```python
from build123d import *

# Parameters (mm, degrees)
CROQUIS1_W              = 440
CROQUIS1_H              = 440
SALIENTE_EXTRUIR1_DEPTH = 9
CROQUIS2_R              = 2
CORTAR_EXTRUIR1_DEPTH   = 312.257128432
CORTAR_EXTRUIR2_DEPTH   = 312.257128432
CORTAR_EXTRUIR3_DEPTH   = 312.257128432
REDONDEO1_R             = 5
CROQUIS5_R              = 2
CORTAR_EXTRUIR4_DEPTH   = 312.257128432
SALIENTE_EXTRUIR3_DEPTH = 9
CROQUIS8_R              = 1.5
CORTAR_EXTRUIR7_DEPTH   = 334.138109498
CROQUIS9_R              = 3
CORTAR_EXTRUIR8_DEPTH   = 334.138109498


with BuildPart() as part:
    # Croquis1 → Saliente-Extruir1 (new body)
    with BuildSketch(Plane(origin=(0, 0, 0), x_dir=(1, 0, 0), z_dir=(0, 1, 0))):
        Rectangle(CROQUIS1_W, CROQUIS1_H)
    extrude(amount=SALIENTE_EXTRUIR1_DEPTH)

    # Croquis2 → Cortar-Extruir1 (cut, through all)
    with BuildSketch(Plane(origin=(0, 9, 0), x_dir=(1, 0, 0), z_dir=(0, 1, 0))):
        with Locations(Location((-210, 210, 0), (0, 0, 270))):
            Circle(CROQUIS2_R)
        with Locations(Location((0, 210, 0), (0, 0, 270))):
            Circle(CROQUIS2_R)
        with Locations(Location((-210, 190, 0), (0, 0, 270))):
            Circle(CROQUIS2_R)
        with Locations(Location((-10, 190, 0), (0, 0, 270))):
            Circle(CROQUIS2_R)
        with Locations(Location((-210, 0, 0), (0, 0, 270))):
            Circle(CROQUIS2_R)
        with Locations(Location((-10, 0, 0), (0, 0, 270))):
            Circle(CROQUIS2_R)
        with Locations(Location((0, -210, 0), (0, 0, 90))):
            Circle(CROQUIS2_R)
        with Locations(Location((-10, -190, 0), (0, 0, 90))):
            Circle(CROQUIS2_R)
        with Locations(Location((-210, -190, 0), (0, 0, 90))):
            Circle(CROQUIS2_R)
        with Locations(Location((-210, -210, 0), (0, 0, 90))):
            Circle(CROQUIS2_R)
        with Locations(Location((10, -190, 0), (0, 0, 270))):
            Circle(CROQUIS2_R)
        with Locations(Location((210, -210, 0), (0, 0, 270))):
            Circle(CROQUIS2_R)
        with Locations(Location((210, -190, 0), (0, 0, 270))):
            Circle(CROQUIS2_R)
        with Locations(Location((210, 0, 0), (0, 0, 90))):
            Circle(CROQUIS2_R)
        with Locations(Location((10, 0, 0), (0, 0, 90))):
            Circle(CROQUIS2_R)
        with Locations(Location((10, 190, 0), (0, 0, 90))):
            Circle(CROQUIS2_R)
        with Locations(Location((210, 190, 0), (0, 0, 90))):
            Circle(CROQUIS2_R)
        with Locations(Location((210, 210, 0), (0, 0, 90))):
            Circle(CROQUIS2_R)
        with Locations(Location((-91.6, 190, 0), (0, 0, 270))):
            Circle(CROQUIS2_R)
        with Locations(Location((91.6, 190, 0), (0, 0, 90))):
            Circle(CROQUIS2_R)
        with Locations(Location((-91.6, 0, 0), (0, 0, 270))):
            Circle(CROQUIS2_R)
        with Locations(Location((91.6, -190, 0), (0, 0, 270))):
            Circle(CROQUIS2_R)
        with Locations(Location((-91.6, -190, 0), (0, 0, 90))):
            Circle(CROQUIS2_R)
        with Locations(Location((91.6, 0, 0), (0, 0, 90))):
            Circle(CROQUIS2_R)
    extrude(amount=-CORTAR_EXTRUIR1_DEPTH, mode=Mode.SUBTRACT)

    # Croquis3 → Cortar-Extruir2 (cut, through all)
    with BuildSketch(Plane(origin=(0, 9, 0), x_dir=(1, 0, 0), z_dir=(0, 1, 0))):
        Polygon((-200, -70), (-200, 70), (-191, 85), (-171, 85), (-162, 70), (-162, -70), (-171, -85), (-191, -85), align=None)
        Polygon((171, 85), (162, 70), (162, -70), (171, -85), (191, -85), (200, -70), (200, 70), (191, 85), align=None)
    extrude(amount=-CORTAR_EXTRUIR2_DEPTH, mode=Mode.SUBTRACT)

    # Croquis4 → Cortar-Extruir3 (cut, through all)
    with BuildSketch(Plane(origin=(0, 9, 0), x_dir=(1, 0, 0), z_dir=(0, 1, 0))):
        with BuildLine():
            Line((160.8, 100), (140.8, 100))
            ThreePointArc((140.8, 100), (112.515728753, 111.715728753), (100.8, 140))
            Line((100.8, 140), (100.8, 160))
            ThreePointArc((100.8, 160), (112.515728753, 188.284271247), (140.8, 200))
            Line((140.8, 200), (160.8, 200))
            ThreePointArc((160.8, 200), (189.084271247, 188.284271247), (200.8, 160))
            Line((200.8, 160), (200.8, 140))
            ThreePointArc((200.8, 140), (189.084271247, 111.715728753), (160.8, 100))
        make_face()
        with BuildLine():
            Line((-160.8, 200), (-140.8, 200))
            ThreePointArc((-140.8, 200), (-112.515728753, 188.284271247), (-100.8, 160))
            Line((-100.8, 160), (-100.8, 140))
            ThreePointArc((-100.8, 140), (-112.515728753, 111.715728753), (-140.8, 100))
            Line((-140.8, 100), (-160.8, 100))
            ThreePointArc((-160.8, 100), (-189.084271247, 111.715728753), (-200.8, 140))
            Line((-200.8, 140), (-200.8, 160))
            ThreePointArc((-200.8, 160), (-189.084271247, 188.284271247), (-160.8, 200))
        make_face()
        with BuildLine():
            Line((-160.8, -100), (-140.8, -100))
            ThreePointArc((-140.8, -100), (-112.515728753, -111.715728753), (-100.8, -140))
            Line((-100.8, -140), (-100.8, -160))
            ThreePointArc((-100.8, -160), (-112.515728753, -188.284271247), (-140.8, -200))
            Line((-140.8, -200), (-160.8, -200))
            ThreePointArc((-160.8, -200), (-189.084271247, -188.284271247), (-200.8, -160))
            Line((-200.8, -160), (-200.8, -140))
            ThreePointArc((-200.8, -140), (-189.084271247, -111.715728753), (-160.8, -100))
        make_face()
        with BuildLine():
            Line((200.8, -160), (200.8, -140))
            ThreePointArc((200.8, -140), (189.084271247, -111.715728753), (160.8, -100))
            Line((160.8, -100), (140.8, -100))
            ThreePointArc((140.8, -100), (112.515728753, -111.715728753), (100.8, -140))
            Line((100.8, -140), (100.8, -160))
            ThreePointArc((100.8, -160), (112.515728753, -188.284271247), (140.8, -200))
            Line((140.8, -200), (160.8, -200))
            ThreePointArc((160.8, -200), (189.084271247, -188.284271247), (200.8, -160))
        make_face()
    extrude(amount=-CORTAR_EXTRUIR3_DEPTH, mode=Mode.SUBTRACT)

    # Redondeo1
    redondeo1_edges = [part.edges().sort_by_distance(p)[0] for p in [
        (-171, 4.5, 85),
        (-191, 4.5, 85),
        (-191, 4.5, -85),
        (-171, 4.5, -85),
        (171, 4.5, -85),
        (191, 4.5, -85),
        (191, 4.5, 85),
        (171, 4.5, 85),
    ]]
    fillet(redondeo1_edges, radius=REDONDEO1_R)

    # Croquis5 → Cortar-Extruir4 (cut, through all)
    with BuildSketch(Plane(origin=(0, 9, 0), x_dir=(1, 0, 0), z_dir=(0, 1, 0))):
        with Locations(Location((-210, 165, 0), (0, 0, 270))):
            Circle(CROQUIS5_R)
        with Locations(Location((-210, 135, 0), (0, 0, 270))):
            Circle(CROQUIS5_R)
        with Locations(Location((-210, -135, 0), (0, 0, 90))):
            Circle(CROQUIS5_R)
        with Locations(Location((-210, -165, 0), (0, 0, 90))):
            Circle(CROQUIS5_R)
        with Locations(Location((210, -165, 0), (0, 0, 270))):
            Circle(CROQUIS5_R)
        with Locations(Location((210, -135, 0), (0, 0, 270))):
            Circle(CROQUIS5_R)
        with Locations(Location((210, 135, 0), (0, 0, 90))):
            Circle(CROQUIS5_R)
        with Locations(Location((210, 165, 0), (0, 0, 90))):
            Circle(CROQUIS5_R)
    extrude(amount=-CORTAR_EXTRUIR4_DEPTH, mode=Mode.SUBTRACT)

    # Croquis7 → Saliente-Extruir3 (add)
    with BuildSketch(Plane(origin=(0, 9, 0), x_dir=(1, 0, 0), z_dir=(0, 1, 0))):
        Polygon((220, 220), (-220, 220), (-190, 250), (190, 250), align=None)
        Polygon((220, -220), (190, -250), (-190, -250), (-220, -220), align=None)
    extrude(amount=-SALIENTE_EXTRUIR3_DEPTH)

    # Croquis8 → Cortar-Extruir7 (cut, through all)
    with BuildSketch(Plane(origin=(0, 9, 0), x_dir=(1, 0, 0), z_dir=(0, 1, 0))):
        with Locations(Location((-75, 242.5, 0), (0, 0, 270))):
            Circle(CROQUIS8_R)
        with Locations(Location((-75, 227.5, 0), (0, 0, 90))):
            Circle(CROQUIS8_R)
        with Locations(Location((75, 227.5, 0), (0, 0, 270))):
            Circle(CROQUIS8_R)
        with Locations(Location((75, 242.5, 0), (0, 0, 90))):
            Circle(CROQUIS8_R)
        with Locations(Location((-186.893398282, 242.5, 0), (0, 0, 270))):
            Circle(CROQUIS8_R)
        with Locations(Location((-204.571067812, 224.82233047, 0), (0, 0, 270))):
            Circle(CROQUIS8_R)
        with Locations(Location((-156.893398282, 242.5, 0), (0, 0, 270))):
            Circle(CROQUIS8_R)
        with Locations(Location((-156.893398282, 227.5, 0), (0, 0, 90))):
            Circle(CROQUIS8_R)
        with Locations(Location((-186.893398282, 227.5, 0), (0, 0, 90))):
            Circle(CROQUIS8_R)
        with Locations(Location((186.893398282, 227.5, 0), (0, 0, 270))):
            Circle(CROQUIS8_R)
        with Locations(Location((156.893398282, 227.5, 0), (0, 0, 270))):
            Circle(CROQUIS8_R)
        with Locations(Location((156.893398282, 242.5, 0), (0, 0, 90))):
            Circle(CROQUIS8_R)
        with Locations(Location((204.571067812, 224.82233047, 0), (0, 0, 90))):
            Circle(CROQUIS8_R)
        with Locations(Location((186.893398282, 242.5, 0), (0, 0, 90))):
            Circle(CROQUIS8_R)
        with Locations(Location((186.893398282, -242.5, 0), (0, 0, 270))):
            Circle(CROQUIS8_R)
        with Locations(Location((204.571067812, -224.82233047, 0), (0, 0, 270))):
            Circle(CROQUIS8_R)
        with Locations(Location((156.893398282, -242.5, 0), (0, 0, 270))):
            Circle(CROQUIS8_R)
        with Locations(Location((156.893398282, -227.5, 0), (0, 0, 90))):
            Circle(CROQUIS8_R)
        with Locations(Location((186.893398282, -227.5, 0), (0, 0, 90))):
            Circle(CROQUIS8_R)
        with Locations(Location((-186.893398282, -227.5, 0), (0, 0, 270))):
            Circle(CROQUIS8_R)
        with Locations(Location((-156.893398282, -227.5, 0), (0, 0, 270))):
            Circle(CROQUIS8_R)
        with Locations(Location((-156.893398282, -242.5, 0), (0, 0, 90))):
            Circle(CROQUIS8_R)
        with Locations(Location((-204.571067812, -224.82233047, 0), (0, 0, 90))):
            Circle(CROQUIS8_R)
        with Locations(Location((-186.893398282, -242.5, 0), (0, 0, 90))):
            Circle(CROQUIS8_R)
    extrude(amount=-CORTAR_EXTRUIR7_DEPTH, mode=Mode.SUBTRACT)

    # Croquis9 → Cortar-Extruir8 (cut, through all)
    with BuildSketch(Plane(origin=(0, 9, 0), x_dir=(1, 0, 0), z_dir=(0, 1, 0))):
        with Locations(Location((-210, 210, 0), (0, 0, 270))):
            Circle(CROQUIS9_R)
        with Locations(Location((-210, 190, 0), (0, 0, 270))):
            Circle(CROQUIS9_R)
        with Locations(Location((-210, 165, 0), (0, 0, 270))):
            Circle(CROQUIS9_R)
        with Locations(Location((-210, 135, 0), (0, 0, 270))):
            Circle(CROQUIS9_R)
        with Locations(Location((-210, 0, 0), (0, 0, 270))):
            Circle(CROQUIS9_R)
        with Locations(Location((-91.6, 0, 0), (0, 0, 270))):
            Circle(CROQUIS9_R)
        with Locations(Location((-10, 0, 0), (0, 0, 270))):
            Circle(CROQUIS9_R)
        with Locations(Location((0, 210, 0), (0, 0, 270))):
            Circle(CROQUIS9_R)
        with Locations(Location((-10, 190, 0), (0, 0, 270))):
            Circle(CROQUIS9_R)
        with Locations(Location((-91.6, 190, 0), (0, 0, 270))):
            Circle(CROQUIS9_R)
        with Locations(Location((210, 0, 0), (0, 0, 90))):
            Circle(CROQUIS9_R)
        with Locations(Location((91.6, 0, 0), (0, 0, 90))):
            Circle(CROQUIS9_R)
        with Locations(Location((10, 0, 0), (0, 0, 90))):
            Circle(CROQUIS9_R)
        with Locations(Location((91.6, 190, 0), (0, 0, 90))):
            Circle(CROQUIS9_R)
        with Locations(Location((10, 190, 0), (0, 0, 90))):
            Circle(CROQUIS9_R)
        with Locations(Location((210, 135, 0), (0, 0, 90))):
            Circle(CROQUIS9_R)
        with Locations(Location((210, 165, 0), (0, 0, 90))):
            Circle(CROQUIS9_R)
        with Locations(Location((210, 190, 0), (0, 0, 90))):
            Circle(CROQUIS9_R)
        with Locations(Location((210, 210, 0), (0, 0, 90))):
            Circle(CROQUIS9_R)
        with Locations(Location((210, -210, 0), (0, 0, 270))):
            Circle(CROQUIS9_R)
        with Locations(Location((210, -190, 0), (0, 0, 270))):
            Circle(CROQUIS9_R)
        with Locations(Location((210, -165, 0), (0, 0, 270))):
            Circle(CROQUIS9_R)
        with Locations(Location((210, -135, 0), (0, 0, 270))):
            Circle(CROQUIS9_R)
        with Locations(Location((10, -190, 0), (0, 0, 270))):
            Circle(CROQUIS9_R)
        with Locations(Location((91.6, -190, 0), (0, 0, 270))):
            Circle(CROQUIS9_R)
        with Locations(Location((-91.6, -190, 0), (0, 0, 90))):
            Circle(CROQUIS9_R)
        with Locations(Location((-10, -190, 0), (0, 0, 90))):
            Circle(CROQUIS9_R)
        with Locations(Location((0, -210, 0), (0, 0, 90))):
            Circle(CROQUIS9_R)
        with Locations(Location((-210, -135, 0), (0, 0, 90))):
            Circle(CROQUIS9_R)
        with Locations(Location((-210, -165, 0), (0, 0, 90))):
            Circle(CROQUIS9_R)
        with Locations(Location((-210, -190, 0), (0, 0, 90))):
            Circle(CROQUIS9_R)
        with Locations(Location((-210, -210, 0), (0, 0, 90))):
            Circle(CROQUIS9_R)
    extrude(amount=-CORTAR_EXTRUIR8_DEPTH, mode=Mode.SUBTRACT)


solid = part.part
```
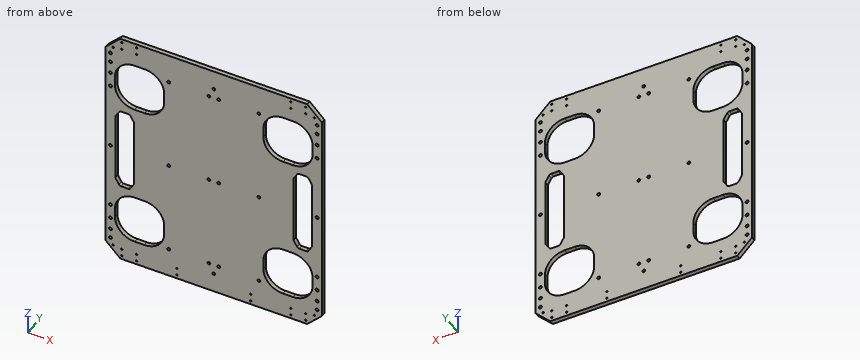
Verification items for the finished model (mm, model axes). Round coordinates to 2 decimals unless told otherwise and drop trailing zeros. Write each loop counter-clockwise with the first axis right and the second up, starting at its lowest first coordinate (ties: lowest second). Pieces come first, ordered by that corner, then holes. Notation, with made-up numbers: (73.25, 9) -> (111.25, 9) arc R26 ccw to (111.25, 33) -> close; hole circle Ø10 at (-27, -14). An arc over 180 degrees is marked (long way). Write each question's results on one line, items separated by ' | '.
Q1. Thickness scan on probe 1 along X at (y, z) = (8.25, 16); probe 2 along X at (y, z) = (4.75, -145); probe 3 along X at (y, z) = (6.5, 227.5). Record the ranges inside material, lowest first.
Derived:
probe 1: x = -220 to -200, -162 to 162, 200 to 220 | probe 2: x = -220 to -200.8, -100.8 to 100.8, 200.8 to 220 | probe 3: x = -212.5 to -188.39, -185.39 to -158.39, -155.39 to 155.39, 158.39 to 185.39, 188.39 to 212.5
Q2. Sectioned sample at B-B, the plane x = -180. Record the boundary of the cut face in (y, z), and give its area (3 significant figures).
Derived:
outline: (0, -250) -> (9, -250) -> (9, -195.09) -> (0, -195.09) -> close; (0, -104.91) -> (9, -104.91) -> (9, -85) -> (0, -85) -> close; (0, 85) -> (9, 85) -> (9, 104.91) -> (0, 104.91) -> close; (0, 195.09) -> (9, 195.09) -> (9, 250) -> (0, 250) -> close | area: 1,350 mm²
Q3. Sectioned sample at A-A, the plane z = 12. Record the boundary of the cut face in (x, y), and give its area (3 significant figures).
Derived:
outline: (-220, 0) -> (-200, 0) -> (-200, 9) -> (-220, 9) -> close; (-162, 0) -> (162, 0) -> (162, 9) -> (-162, 9) -> close; (200, 0) -> (220, 0) -> (220, 9) -> (200, 9) -> close | area: 3,280 mm²
Q4. Go/stop test with flat-tipped pins: pin 1 Ø5 at (x, z) = (156.89, -227.5) entering from +Y; pin 2 Ø3.5 at (x, z) = (-210, -165) entering from -Y. Record where each tip stops, or that it passes through.
Derived:
pin 1: stops at y = 9 | pin 2: passes through
Q5. Sectioned sample at C-C, the plane y = 7. Give the number of separate pieces and of enclosed holes in the cut face, and give its area (3 significant figures).
Derived:
separate pieces: 1 | enclosed holes: 62 | area: 170,000 mm²
